from build123d import *

# Parameters (mm, degrees)
F1_DEPTH = 25.4


with BuildPart() as f1:
    # F0 (on Front) → F1 (new body)
    with BuildSketch(Plane.XZ):
        with BuildLine():
            ThreePointArc((-16.513216, 43.049148), (-26.195994, 36.279159), (-26.559999, 24.469991))
            ThreePointArc((-26.559999, 24.469991), (-23.612281, 22.442675), (-21.448272, 19.593795))
            ThreePointArc((-21.448272, 19.593795), (-21.165753, 19.026637), (-20.915549, 18.444501))
            ThreePointArc((-20.915549, 18.444501), (-20.912799, 18.437567), (-20.910054, 18.430631))
            ThreePointArc((-20.910054, 18.430631), (-21.318885, 18.566069), (-21.724175, 18.711757))
            ThreePointArc((-21.724175, 18.711757), (-22.174114, 13.422676), (-20.669998, 8.332051))
            ThreePointArc((-20.669998, 8.332051), (-23.018125, 7.130784), (-25.1052, 5.518067))
            ThreePointArc((-25.1052, 5.518067), (-15.529674, -8.146325), (-4.646679, 4.50147))
            ThreePointArc((-4.646679, 4.50147), (7.250734, 11.666572), (4.286682, 25.234973))
            ThreePointArc((4.286682, 25.234973), (1.349789, 25.007459), (-1.593968, 25.114212))
            ThreePointArc((-1.593968, 25.114212), (-2.619774, 23.756453), (-3.775427, 22.507351))
            ThreePointArc((-3.775427, 22.507351), (-2.980585, 23.809554), (-2.341596, 25.194905))
            ThreePointArc((-2.341596, 25.194905), (-3.060024, 25.293199), (-3.775427, 25.411526))
            ThreePointArc((-3.775427, 25.411526), (-3.329014, 26.854447), (-2.799791, 28.269095))
            ThreePointArc((-2.799791, 28.269095), (-5.177523, 28.210416), (-7.496269, 27.680819))
            ThreePointArc((-7.496269, 27.680819), (-5.112054, 31.158026), (-2.073727, 34.081041))
            ThreePointArc((-2.073727, 34.081041), (-7.654003, 41.204792), (-16.513216, 43.049148))
        make_face()
    extrude(amount=F1_DEPTH)


solid = f1.part
For this review, take the finished solid that the model builds, in its own axes (mm). A direction names the side the tool comes from. Round coordinates to 2 decimals unless told otherwise and drop trailing zeros. Write each loop counter-clockwise with the first axis right and the second up, starting at its lowest first coordinate (ties: lowest second). Pieces come first, ordered by that corner, then holes. Notation, with made-up numbers: M -39.75,33.5 L 19.25,33.5 A25 ccw 19.25,61.5 Z; hole C 30,40.5 d3. An arc over 180 degrees is marked long. Write item = value, one per line. Start each with the question number.
(1) We need section C-C (z = 7). Give the boundary of the cut face in (x, y), then the cut area to 3 significant figures.
(2) The part is to be moulded in two halves that separate along X. For faces 3 (the face through (-22.18, -12.52, 13.5)), 4 (the face through (-10, 0, 18)), 5 (the face through (1.39, -12.52, 25.01)), 6 (the face through (-5.144, -12.522, 28.215)), say which applies: +X half, -X half, draft (parallel to the pull), parting line (faces both ways), or undercut.
(3) Clearance check with flat-ended pins moving along their axes: pin 1 Ø8 at (x, y) = (-7.5, -9) entering from +Z; pin 2 Ø12 at (x, y) = (4, -18) entering from -Z; pin 3 Ø6 at (y, z) = (-16.5, 24.5) entering from -X. State where each tip first meets the part, or that it passes through.
(4) For line 1 along Z through (x, y) = (-22.5, -10); line 2 along X through (y, z) = (-22, 23); line 3 along Z through (x, y) = (-15, -16), list the stretches that pass through material, from the lowest coordinate up.
(5) For faces 1 (the face through (-22.99, -12.52, 7.15)), 2 (the face through (-10, -25.4, 18)), list the 3-axis set-ups (+Z, -Z, +X, -X, +Y, -Y) from which the entire face can be reached by the end or side of a thin tool; tool diameter is ignored.
(6) We need section A-A (x = -24). Give the boundary of the cut face in (y, z), then the cut area to 3 significant figures.
(7) We need section D-D (x = 2). Give the boundary of the cut face in (y, z), then the cut area to 3 significant figures.
Results found:
q1.outline = M -23.22,-25.4 L 3.65,-25.4 L 3.65,0 L -23.22,0 Z
q1.area = 683 mm²
q2.face_3 = -X half
q2.face_4 = draft
q2.face_5 = undercut
q2.face_6 = undercut
q3.pin_1 = 42.82
q3.pin_2 = 4.58
q3.pin_3 = -27.54
q4.line_1 = -5.04 to 7.44, 21.21 to 40.56
q4.line_2 = -24.24 to -3.45, -3.29 to 6.22
q4.line_3 = -8.16 to 43.18
q5.face_1 = -X, +Y, -Y
q5.face_2 = +Z, -Z, +X, -X, -Y
q6.outline = M -25.4,-3.14 L 0,-3.14 L 0,6.45 L -25.4,6.45 Z; M -25.4,22.8 L 0,22.8 L 0,39.25 L -25.4,39.25 Z
q6.area = 661 mm²
q7.outline = M -25.4,5.91 L 0,5.91 L 0,25.03 L -25.4,25.03 Z
q7.area = 486 mm²
